Source: three-view drawing plus pictorial views. Frame: mm from the lowest corner of the part. Give positions to 0.01 mm unless a question says otherwise; leave off trailing zeros. Write each loop counter-clockwise with the first axis right and the second up, starting at its lowest first coordinate (ties: lowest second). Pieces come first, ordered by that corner, then holes. Notation, with made-up numbers: (71, 3) -> (93, 3) arc R9 ccw to (93, 7) -> close; hole circle Ø2 at (10, 75). An arc over 180 degrees is marked (long way). Use a Markdown table: item, result. Add a question column.
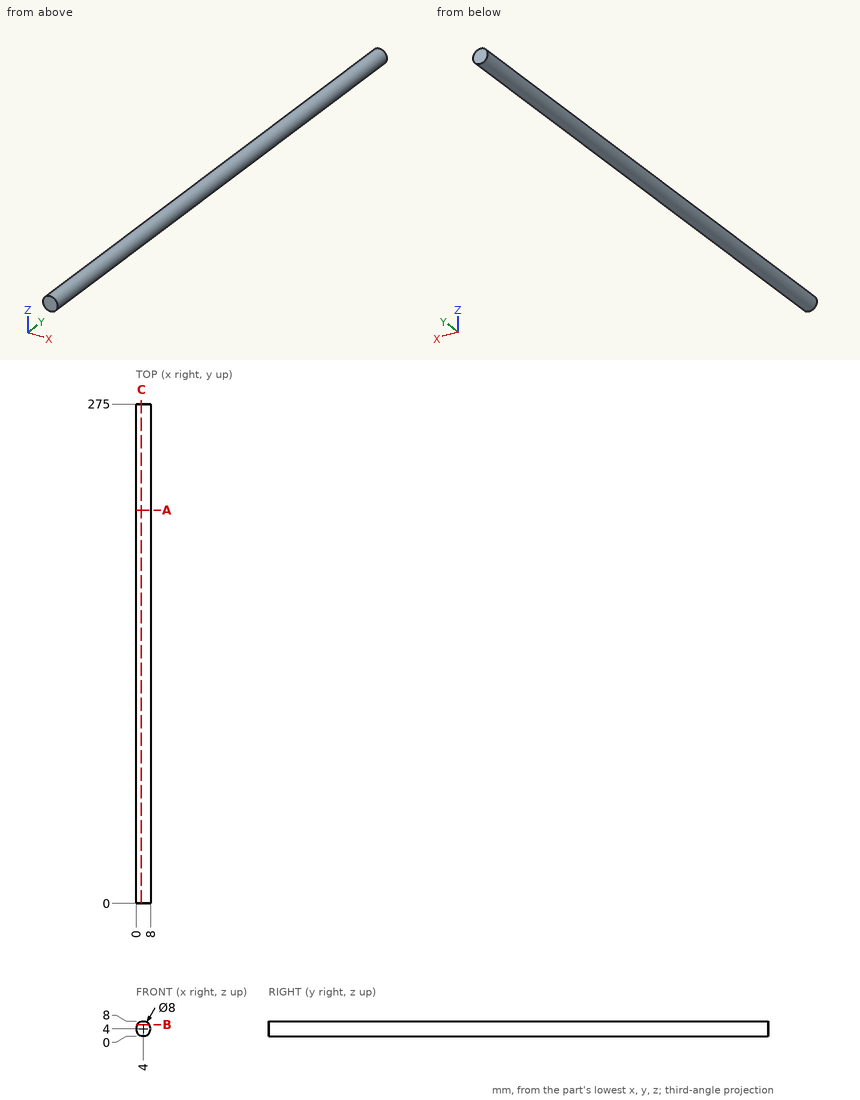
(1) Material intervals for L1, parallel to Z at x = 5.5, y = 262; L2, parallel to X at y = 40, z = 3.25, sorted ascending.
(2) First-contact query: pin 1 Ø1.5 at (x, y) = (7, 119.5) entering from +Z; pin 2 Ø3 at (x, y) = (6, 162) entering from +Z. Flat tips, straight axial feed; report the tip coordinate or a pass-through.
(3) Cut plane C-C on x = 3. Return the cut outline in (y, z).
(4) Cut plane A-A on y = 216.5. Return the cut outline in (x, z), then the cut area to 3 significant figures.
(5) Cut plane B-B on z = 6.25. Return the cut outline in (x, y), then the cut area to 3 significant figures.
Output:
| question | item | result |
|---|---|---|
| 1 | L1 | 0.29 to 7.71 |
| 1 | L2 | 0.07 to 7.93 |
| 2 | pin 1 | z = 7.31 |
| 2 | pin 2 | z = 7.97 |
| 3 | outline | (0, 0.13) -> (275, 0.13) -> (275, 7.87) -> (0, 7.87) -> close |
| 4 | outline | circle Ø8 at (4, 4) |
| 4 | area | 50.3 mm^2 |
| 5 | outline | (0.69, 0) -> (7.31, 0) -> (7.31, 275) -> (0.69, 275) -> close |
| 5 | area | 1,820 mm^2 |
